Check sheet for the modelled part. Datum: model origin and axes. Units: mm. Face numbers are marked on the shaded views. A direction names the side the tool comes from. Give positions to 0.01 mm unless a question says otherwise; leave off trailing zeros. Write each loop counter-clockwise with the first axis right and the second up, starting at its lowest first coordinate (ties: lowest second). Pieces come first, ordered by that corner, then holes. Notation, with made-up numbers: (30.5, 5) -> (88.5, 5) arc R20 ccw to (88.5, 21) -> close; hole circle Ø11 at (86, 2). An arc over 180 degrees is marked (long way). Use a Markdown table: item, result. Add a question column.
1. Set-up check for the marked faces 1, 2 and 3: record each of +Z, -Z, +X, -X, +Y, -Y from which the full face is reachable in a straight line by a thin tool's end or side.
2. Cross-section at A-A (y = 14). Enter the section's corners in (x, z).
3. Release check for a two-part mould opening along X. For the marked faces 4 and 5 record: released by +X, released by -X, zero draft, split by the parting line, or undercut.
4. Cross-section at B-B (z = 0). Enter the section's corners in (x, y).
5. Cross-section at D-D (x = -18). Enter the section's corners in (y, z).
6. Gauge pin test, flat ends, axial feed: P1, Ø2, axis at y = 39.5, z = -0.5, coming from the +X side; P2, Ø5, axis at x = -30, z = 3.5, coming from the +Y side; P3, Ø0.6, axis at y = 39.5, z = -5, coming from the -X side. Record the tip position at first contact, or that the pin passes through.
7. Cross-section at C-C (z = -20). Enter the section's corners in (x, y), then the cut area to 3 significant figures.
8. Scan lines: probe 1 along Z at (x, y) = (-21, -2); probe 2 along Y at (x, z) = (-13.5, -5.5); probe 3 along Z at (x, y) = (0, -39.5). Record each from-to range of solid material in increasing order. Write a range as [from, to].
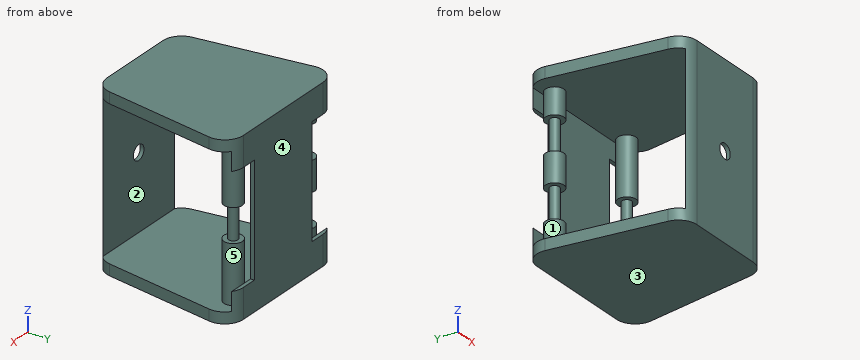
from build123d import *

# Parameters (mm, degrees)
BOSS_EXTRUDE1_DEPTH = 46
SKETCH4_W           = 80
SKETCH4_H           = 76
CUT_EXTRUDE1_DEPTH  = 46
SKETCH5_R           = 5
BOSS_EXTRUDE2_DEPTH = 8
SKETCH6_R           = 2.5
BOSS_EXTRUDE3_DEPTH = 18
SKETCH8_R           = 2.5
BOSS_EXTRUDE4_DEPTH = 18
SKETCH9_R           = 5
BOSS_EXTRUDE5_DEPTH = 14
BOSS_EXTRUDE6_START = 14
SKETCH10_R          = 5
BOSS_EXTRUDE6_DEPTH = 14
SKETCH11_R          = 2.5
BOSS_EXTRUDE7_DEPTH = 9
SKETCH12_R          = 5
BOSS_EXTRUDE8_DEPTH = 31
BOSS_EXTRUDE9_START = 31
SKETCH13_R          = 5
BOSS_EXTRUDE9_DEPTH = 31
SKETCH14_W          = 20
SKETCH14_H          = 60
CUT_EXTRUDE2_DEPTH  = 2.2
FILLET1_R           = 10
FILLET2_R           = 10
SKETCH15_R          = 4
CUT_EXTRUDE3_DEPTH  = 2.2


with BuildPart() as part:
    # Sketch3 → Boss-Extrude1 (new, symmetric)
    with BuildSketch(Plane.XY):
        Polygon((42, 40), (-42, 40), (-30, -40), (30, -40), align=None)
    extrude(amount=BOSS_EXTRUDE1_DEPTH, both=True)

    # Sketch4 → Cut-Extrude1 (cut, symmetric)
    with BuildSketch(Plane(origin=(0, 0, 0), x_dir=(0, 0, -1), z_dir=(1, 0, 0))):
        Rectangle(SKETCH4_W, SKETCH4_H)
    extrude(amount=CUT_EXTRUDE1_DEPTH, both=True, mode=Mode.SUBTRACT)



with BuildPart() as body_2:
    # Sketch5 → Boss-Extrude2 (new, symmetric)
    with BuildSketch(Plane.XY):
        with Locations((-27.5, 32.5)):
            Circle(SKETCH5_R)
    extrude(amount=BOSS_EXTRUDE2_DEPTH, both=True)

    # Sketch6 → Boss-Extrude3 (add)
    with BuildSketch(Plane.XY.offset(8)):
        with Locations((-27.5, 32.5)):
            Circle(SKETCH6_R)
    extrude(amount=BOSS_EXTRUDE3_DEPTH)

    # Sketch8 → Boss-Extrude4 (add)
    with BuildSketch(Plane(origin=(0, 0, -8), x_dir=(-1, 0, 0), z_dir=(0, 0, -1))):
        with Locations(Location((27.5, 32.5, 0), (0, 0, 180))):
            Circle(SKETCH8_R)
    extrude(amount=BOSS_EXTRUDE4_DEPTH)


with BuildPart() as part_1:
    add(part.part)

    add(body_2.part)  # Boss-Extrude5 merges body 2
    # Sketch9 → Boss-Extrude5 (add)
    with BuildSketch(Plane(origin=(0, 0, -26), x_dir=(-1, 0, 0), z_dir=(0, 0, -1))):
        with Locations(Location((27.5, 32.5, 0), (0, 0, 180))):
            Circle(SKETCH9_R)
    extrude(amount=BOSS_EXTRUDE5_DEPTH)

    # Sketch10 → Boss-Extrude6 (add)
    with BuildSketch(Plane.XY.offset(26).offset(BOSS_EXTRUDE6_START)):
        with Locations((-27.5, 32.5)):
            Circle(SKETCH10_R)
    extrude(amount=-BOSS_EXTRUDE6_DEPTH)



with BuildPart() as body_2_2:
    # Sketch11 → Boss-Extrude7 (new, symmetric)
    with BuildSketch(Plane.XY):
        with Locations((27.5, 32.5)):
            Circle(SKETCH11_R)
    extrude(amount=BOSS_EXTRUDE7_DEPTH, both=True)


with BuildPart() as part_2:
    add(part_1.part)

    add(body_2_2.part)  # Boss-Extrude8 merges body 2 2
    # Sketch12 → Boss-Extrude8 (add)
    with BuildSketch(Plane.XY.offset(9)):
        with Locations(Location((27.5, 32.5, 0), (0, 0, 180))):
            Circle(SKETCH12_R)
    extrude(amount=BOSS_EXTRUDE8_DEPTH)

    # Sketch13 → Boss-Extrude9 (add)
    with BuildSketch(Plane(origin=(0, 0, -9), x_dir=(-1, 0, 0), z_dir=(0, 0, -1)).offset(BOSS_EXTRUDE9_START)):
        with Locations((-27.5, 32.5)):
            Circle(SKETCH13_R)
    extrude(amount=-BOSS_EXTRUDE9_DEPTH)

    # Sketch14 → Cut-Extrude2 (cut)
    with BuildSketch(Plane(origin=(0, 40, 0), x_dir=(1, 0, 0), z_dir=(0, 1, 0))):
        with Locations((32, 0)):
            Rectangle(SKETCH14_W, SKETCH14_H)
        with Locations((-32, 0)):
            Rectangle(SKETCH14_W, SKETCH14_H)
    extrude(amount=-CUT_EXTRUDE2_DEPTH, mode=Mode.SUBTRACT)

    # Fillet1
    fillet1_edges = [part_2.edges().sort_by_distance(p)[0] for p in [
        (42, 40, 38),
        (-42, 40, 38),
        (-42, 40, -38),
        (42, 40, -38),
    ]]
    fillet(fillet1_edges, radius=FILLET1_R)

    # Fillet2
    # the kernel refuses this fillet: 10 mm, written as the material it takes off along each edge
    with BuildSketch(Plane(origin=(-30, -40, -67.52968552), x_dir=(-0.1483404529302443, 0.9889363528682976, 0), z_dir=(0, 0, 1)), Plane(origin=(30, -40, 67.52968552), x_dir=(0.14834045293024473, 0.9889363528682976, 0), z_dir=(0, 0, -1))) as fillet2_piece_1:
        with BuildLine():
            CenterArc((FILLET2_R * 0.861187420808, -FILLET2_R), FILLET2_R, 90, 81.46923439)
            Line((-FILLET2_R * 0.12774893206, -FILLET2_R * 0.85165954707), (0, 0))
            Line((0, 0), (FILLET2_R * 0.861187420808, 0))
        make_face()
    extrude(amount=135.05937104, mode=Mode.SUBTRACT)

    # Sketch15 → Cut-Extrude3 (cut)
    with BuildSketch(Plane.XZ.offset(40)):
        Circle(SKETCH15_R)
    extrude(amount=-CUT_EXTRUDE3_DEPTH, mode=Mode.SUBTRACT)


solid = part_2.part
Worked answers:
| question | item | result |
|---|---|---|
| 1 | face 1 | none |
| 1 | face 2 | +X, -X |
| 1 | face 3 | -Z, +X, -X, +Y, -Y |
| 2 | outline | (-38.1, -46) -> (38.1, -46) -> (38.1, -40) -> (-38.1, -40) -> close; (-38.1, 40) -> (38.1, 40) -> (38.1, 46) -> (-38.1, 46) -> close |
| 3 | face 4 | zero draft |
| 3 | face 5 | undercut |
| 4 | outline | circle Ø10 at (-27.5, 32.5); (-27.39, -38) arc R10 ccw to (-21.39, -40) -> (-4, -40) -> (-4, -38) -> close; (-22, 38) -> (22, 38) -> (22, 40) -> (-22, 40) -> close; (4, -40) -> (21.39, -40) arc R10 ccw to (27.39, -38) -> (4, -38) -> close; circle Ø5 at (27.5, 32.5) |
| 5 | outline | (-40, -46) -> (40, -46) -> (40, 46) -> (-40, 46) -> close; hole (-38, -40) -> (38, -40) -> (38, 40) -> (-38, 40) -> close |
| 6 | P1 | stops at x = 22 |
| 6 | P2 | stops at y = 37.5 |
| 6 | P3 | stops at x = -22 |
| 7 | outline | circle Ø5 at (-27.5, 32.5); (-27.39, -38) arc R10 ccw to (-21.39, -40) -> (21.39, -40) arc R10 ccw to (27.39, -38) -> close; (-22, 38) -> (22, 38) -> (22, 40) -> (-22, 40) -> close; circle Ø10 at (27.5, 32.5) |
| 7 | area | 288 mm² |
| 8 | probe 1 | z = [-46, -40], [40, 46] |
| 8 | probe 2 | y = [-40, -38], [38, 40] |
| 8 | probe 3 | z = [-46, -4], [4, 46] |
